Source: CAD feature listing. Evaluate the final solid. Frame: model axes, mm. Face numbers are marked on the shaded views. A direction names the side the tool comes from. Round coordinates to 2 decimals unless told otherwise and drop trailing zeros. Order: outer loops, then holes, each group sorted by start corner. A loop starts at its lowest first (then second) coordinate and runs counter-clockwise, first axis right, second up. Notation, with made-up numbers: (57.5, 78.5) -> (68.5, 78.5) arc R27 cw to (68.5, 97.5) -> close; hole circle Ø11 at (-33, 15). An arc over 180 degrees is marked (long way). Answer as CSV lines item,"result". Start each with the question number.
(1) Section query C-C (z = -18.75). Output: boundary loops of the cut face in (x, y), plus the area to 3 significant figures.
(2) Pull-direction query (Z, two-part tool) for the marked faces 1, 2, 3 and 4; classes: +Z half, -Z half, draft (parallel to the pull), parting line (faces both ways), or undercut.
(3) Section query B-B (y = -1.7). Output: boundary loops of the cut face in (x, z).
(4) Line query: line 1 along Y through (x, z) = (6, -5.5); line 2 along Z through (x, y) = (35.5, -1.05); line 3 along Z through (x, y) = (34.5, -2.6). Output: solid intervals per line, ascending. Write a range as from..to.
(5) Section query A-A (x = 22). Output: boundary loops of the cut face in (y, z).
(6) Section query D-D (x = 43). Output: boundary loops of the cut face in (y, z), plus the area to 3 significant figures.
(7) Set-up query: the marked faces 5 and 6. Return all of +Z, -Z, +X, -X, +Y, -Y with unobstructed straight access to the full face (end or side cutting, diameter ignored); none if empty.
(8) Contact query for flat-ended pins moving along their axis: P1, Ø1.5, axis at y = -2.5, z = -8.5, coming from the -X side; P2, Ø8, axis at x = 6.5, z = -14.5, coming from the -Y side; P3, Ø6, axis at x = 29, z = -11, coming from the -Y side; P4, Ø1.5, axis at x = 40, y = -2, coming from the +Z side. Output: stop coordinate, or through.
Autodesk Inventor part; units mm, degrees
ref_plane "Work Plane1" through (36, 0.5, -6) normal (0, -1, 0) x (-1, 0, 0)
ref_plane "YZ Plane" through (0, 0, 0) normal (1, 0, 0) x (0, 1, 0)
ref_plane "XZ Plane" through (0, 0, 0) normal (0, 1, 0) x (-1, 0, 0)
sketch "Sketch1" plane through (0, 0, 0) normal (0, 1, 0) x (-1, 0, 0)
  line L0 (0, 0) -> (-50, 0)
  line L1 (-50, 0) -> (-50, -20)
  line L2 (-50, -20) -> (0, -20)
  line L3 (0, -20) -> (0, 0)
  dimension "d0" = 50
  dimension "d1" = 20
extrude "Plate1" add sketch "Sketch1" along normal blind 0.5
sketch "Sketch2" plane through (0, 0.5, 0) normal (0, 1, 0) x (1, 0, 0)
  line L0 (14, 10) -> (36, 10) construction
  line L1 (14, 14) -> (36, 14)
  line L2 (36, 6) -> (14, 6)
  arc A0 (14, 14) -> (14, 6) centre (14, 10) ccw
  arc A1 (36, 6) -> (36, 14) centre (36, 10) ccw
  line L3 (0, 0) -> (0, 20)
  line L4 (50, 0) -> (0, 0)
  point P0 (25, 10)
  point P1 (40, 10)
  point P2 (10, 10)
  dimension "d3" = 8
  dimension "d4" = 30
  dimension "d5" = 25
  dimension "d6" = 10
extrude "Extrusion1" cut sketch "Sketch2" against normal blind 0.5
ref_plane "Work Plane1" through (36, 0.5, -6) normal (0, -1, 0) x (-1, 0, 0)
sketch "Sketch3" plane through (36, 0.5, -6) normal (0, -1, 0) x (-1, 0, 0)
  line L0 (0, 0) -> (22, 0) construction
  arc A0 (22, 0) -> (22, 8) centre (22, 4) ccw construction
  arc A1 (0, 8) -> (0, 0) centre (0, 4) ccw construction
  line L1 (22, 4) -> (0, 4) construction
  line L2 (26, 4) -> (-4, 4)
  arc A2 (22, 0) -> (26, 4) centre (22, 4) ccw
  arc A3 (0, 8) -> (0, 0) centre (0, 4) ccw
  line L3 (22, 0) -> (0, 0)
  arc A4 (-4, 4) -> (0, 0) centre (0, 4) ccw
  line L4 (26, 4) -> (26.5, 4)
  arc A5 (22, -0.5) -> (26.5, 4) centre (22, 4) ccw
  line L5 (22, -0.5) -> (0, -0.5)
  arc A6 (-4.5, 4) -> (0, -0.5) centre (0, 4) ccw
  line L6 (-4, 4) -> (-4.5, 4)
  point P0 (36, -6)
  dimension "d9" = 0.5
revolve "Revolution1" add sketch "Sketch3" angle 180 about axis through (10, 0.5, -10) along (1, 0, 0) contours L4 A5 L5 A6 L6 A3 L3 A2
fillet "Fillet1" radius 2 10 edges at (38.8284, 0.5, -7.1716) (38.8284, 0.5, -12.8284) (25, 0.5, -6) (25, 0.5, -14) (11.1716, 0.5, -7.1716) (11.1716, 0.5, -12.8284) (40.4721, 0, -10) (25, 0, -5.5279) (25, 0, -14.4721) (9.5279, 0, -10)
equation "\"d7\" = Thickness"
equation "\"d9\" = Thickness"
equation "\"d2\" = Thickness"
equation "\"BendRadius\" = Thickness"
equation "\"BendReliefWidth\" = Thickness"
equation "\"BendReliefDepth\" = 0.5 * Thickness"
equation "\"CornerReliefSize\" = 4 * Thickness"
equation "\"MinimumRemnant\" = 2 * Thickness"
equation "\"TransitionRadius\" = BendRadius"
equation "\"JacobiRadiusSize\" = BendRadius"
equation "\"GapSize\" = Thickness"
properties part number "CE-4.1.4"
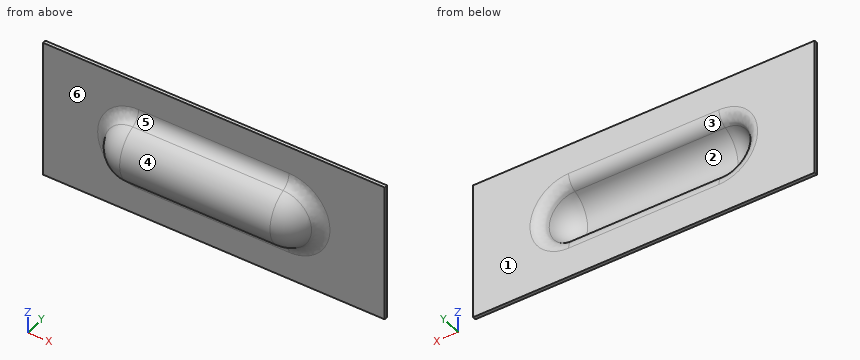
Answer block:
1,outline,"(0, 0) -> (50, 0) -> (50, 0.5) -> (0, 0.5) -> close"
1,area,"25.0 mm2"
2,face 1,"draft"
2,face 2,"undercut"
2,face 3,"undercut"
2,face 4,"parting line"
3,outline,"(14, -13.93) -> (36, -13.93) arc R3.93 ccw to (36, -6.07) -> (14, -6.07) arc R3.93 ccw to start; hole (14, -13.34) -> (36, -13.34) arc R3.34 ccw to (36, -6.66) -> (14, -6.66) arc R3.34 ccw to start"
4,line 1,"0..0.5"
4,line 2,"-14.24..-13.69, -6.31..-5.76"
4,line 3,"-13.26..-12.53, -7.47..-6.74"
5,outline,"(-1.23, -14.15) arc R2 cw to (0, -16) -> (0, -20) -> (0.5, -20) -> (0.5, -15.66) arc R2 ccw to (-0.83, -13.77) arc R4 cw to (-0.83, -6.23) arc R2 ccw to (0.5, -4.34) -> (0.5, 0) -> (0, 0) -> (0, -4) arc R2 cw to (-1.23, -5.85) arc R4.5 ccw to start"
6,outline,"(0, -20) -> (0.5, -20) -> (0.5, 0) -> (0, 0) -> close"
6,area,"10.0 mm2"
7,face 5,"+Z, +X, -X, -Y"
7,face 6,"-Y"
8,P1,"x = 10.33"
8,P2,"y = -0.44"
8,P3,"y = -4"
8,P4,"z = -7.88"
